Autodesk Inventor part; units mm, degrees
ref_plane "Work Plane3" through (0, 0, 40.5) normal (0, 0, 1) x (1, 0, 0)
ref_plane "YZ Plane" through (0, 0, 0) normal (1, 0, 0) x (0, 1, 0)
ref_plane "XZ Plane" through (0, 0, 0) normal (0, 1, 0) x (-1, 0, 0)
sketch "Sketch5" plane through (0, 0, 0) normal (0, 0, 1) x (1, 0, 0)
  line L0 (0, 0) -> (3, 0)
  line L1 (3, 0) -> (3, 51)
  line L2 (3, 51) -> (-110, 51)
  line L3 (-110, 51) -> (-110, 48)
  line L4 (-110, 48) -> (0, 48)
  line L5 (0, 48) -> (0, 0)
  dimension "d32" = 3
  dimension "d33" = 3
  dimension "d34" = 110
  dimension "d35" = 51
extrude "Extrusion4" add sketch "Sketch5" along normal blind 81
sketch "Sketch6" plane through (-110, 48, 0) normal (-1, 0, 0) x (0, 0, 1)
  line L0 (0, 0) -> (81, 0)
  line L1 (0, 3) -> (81, 3)
  line L2 (30.5, 0) -> (50.5, 0)
  line L3 (50.5, 0) -> (50.5, 3)
  line L4 (50.5, 3) -> (30.5, 3)
  line L5 (30.5, 3) -> (30.5, 0)
  point P0 (0, -48)
  point P1 (30.5, 3)
  dimension "d38" = 20
  dimension "d39" = 30.5
extrude "Extrusion5" add sketch "Sketch6" along normal blind 4
sketch "Sketch11" plane through (0, 0, 0) normal (-1, 0, 0) x (0, 0, 1)
  line L0 (81, 0) -> (81, 51)
  line L1 (78, 26) -> (74, 26)
  line L2 (74, 26) -> (74, 16)
  line L3 (74, 16) -> (77, 16)
  line L4 (0, 0) -> (81, 0)
  line L5 (78, 26) -> (78, 16)
  line L6 (81, 48) -> (81, 0)
  line L7 (78, 16) -> (77, 16)
  point P0 (81, 26)
  point P1 (81, 16)
  dimension "d82" = 4
  dimension "d83" = 10
  dimension "d84" = 16
  dimension "d85" = 74
extrude "Extrusion6" add sketch "Sketch11" along normal blind 15
ref_plane "Work Plane3" through (0, 0, 40.5) normal (0, 0, 1) x (1, 0, 0)
mirror "Mirror4" about plane through (0, 0, 40.5) normal (0, 0, 1) of "Extrusion6"
sketch "Sketch15" plane through (0, 16, 74) normal (0, -1, 0) x (1, 0, 0)
  line L0 (0, 4) -> (-15, 4)
  line L1 (-15, 4) -> (-13.3218, 6)
  line L2 (-13.3218, 6) -> (-11.6782, 6)
  line L3 (-11.6782, 6) -> (-10, 4)
  line L4 (-15, 0) -> (-15, 4)
  line L5 (-15, 4) -> (-10, 4)
  line L6 (0, -74) -> (0, 7)
  dimension "d86" = 10
  dimension "d87" = 50
  dimension "d88" = 50
  dimension "d89" = 2
extrude "Extrusion10" add sketch "Sketch15" against normal up to surface (10 mm away)
mirror "Mirror8" about plane through (0, 0, 40.5) normal (0, 0, 1) of "Extrusion10"
properties part number "top"
Part model, mm, in its own coordinate system. A direction names the side the tool comes from. Coordinates: 2 decimals unless noted, no trailing zeros. Order: outer loops, then holes, each group sorted by start corner. A loop starts at its lowest first (then second) coordinate and runs counter-clockwise, first axis right, second up. Notation, with made-up numbers: M -32.5,35 L -18.5,35 A18 cw -18.5,55 Z; hole C -33,-38 d6. An arc over 180 degrees is marked long. Use a Markdown table: item, result.
(1) Cut at C-C on x = -63. Write the cut outline in (y, z).
A:
| item | result |
|---|---|
| outline | M 48,0 L 51,0 L 51,81 L 48,81 Z |
(2) Probe L1, parallel to X at y = 16.5, z = 68; L2, parallel to Y at x = -17.5, z = 77. List the from-to ranges inside material, lowest first.
A:
| item | result |
|---|---|
| L1 | x = 0 to 3 |
| L2 | y = 48 to 51 |
(3) Pull direction Y, two halves, no side cores. Call faces 4 (the flat face through (1, 0, 40)), 5 (the flat face through (-7, 26, 5)), 6 (the flat face through (-55, 51, 40)), 7 (the flat face through (3, 25, 40)): released by +Y, released by -Y, zero draft, split by the parting line, or undercut.
A:
| item | result |
|---|---|
| face 4 | released by -Y |
| face 5 | undercut |
| face 6 | released by +Y |
| face 7 | zero draft |
(4) Cut at D-D on z = 23. Write the cut outline in (x, y).
A:
| item | result |
|---|---|
| outline | M -110,48 L 0,48 L 0,0 L 3,0 L 3,51 L -110,51 Z |
(5) Cut at B-B on z = 48. Write the cut outline in (x, y).
A:
| item | result |
|---|---|
| outline | M -114,48 L 0,48 L 0,0 L 3,0 L 3,51 L -114,51 Z |
(6) Tool access for faces 1 (the flat face through (-5, 21, 78)), 2 (the flat face through (-8, 16, 76)), 3 (the flat face through (-110, 50, 66)): list every direction of +Z, -Z, +X, -X, +Y, -Y with a clear straight run to the whole face (end or side of a thin tool).
A:
| item | result |
|---|---|
| face 1 | +Z, -Y |
| face 2 | +Z, -Z, -X, -Y |
| face 3 | +Z, -X, +Y, -Y |
(7) Cut at A-A on y = 18. Write the cut outline in (x, z).
A:
| item | result |
|---|---|
| outline | M -15,3 L -13.32,1 L -11.68,1 L -10,3 L 0,3 L 0,0 L 3,0 L 3,81 L 0,81 L 0,78 L -10,78 L -11.68,80 L -13.32,80 L -15,78 L -15,74 L 0,74 L 0,7 L -15,7 Z |
(8) Flat gauge pins, fed straight in: pin 1 (1.2 mm diameter, centred on y = 20.5, z = 76.5, fed in from -X); pin 2 (24 mm diameter, centred on y = 24.5, z = 57.5, fed in from -X); pin 3 (2.5 mm diameter, centred on y = 50, z = 16.5, fed in from -X). Where does each tip first touch, or does it go through?
A:
| item | result |
|---|---|
| pin 1 | stops at x = -15 |
| pin 2 | stops at x = 0 |
| pin 3 | stops at x = -110 |
